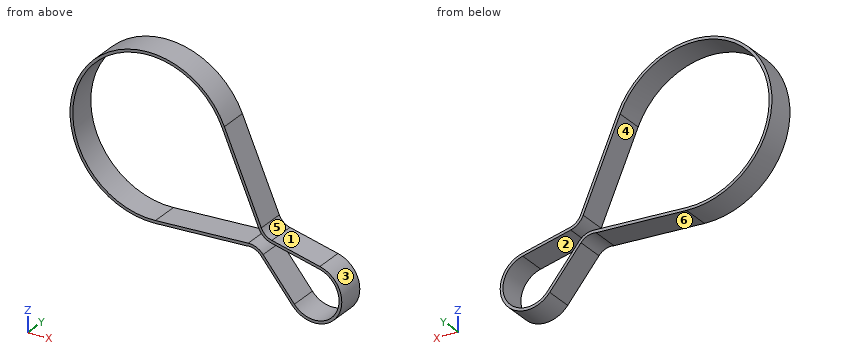
from build123d import *

# Parameters (mm, degrees)
BOSS_EXTRUDE1_DEPTH = 7
BOSS_EXTRUDE2_DEPTH = 3


with BuildPart() as part:
    # Sketch1 → Boss-Extrude1 (new body)
    with BuildSketch(Plane(origin=(0, 0, 0), x_dir=(1, 0, 0), z_dir=(0, 1, 0))):
        with BuildLine():
            Line((29.22824924, 30.681159688), (17.850659856, 16.897054356))
            ThreePointArc((17.850659856, 16.897054356), (15.379675631, 15.1910369), (12.380917697, 15.03705815))
            Line((12.380917697, 15.03705815), (-20.537634361, 17.060906053))
            ThreePointArc((-20.537634361, 17.060906053), (-47.281869491, -27.461627718), (4.525488573, -23.786335009))
            Line((4.525488573, -23.786335009), (17.958953394, 7.231589211))
            ThreePointArc((17.958953394, 7.231589211), (19.505297976, 9.287886756), (21.817685297, 10.415896524))
            Line((21.817685297, 10.415896524), (39.268754989, 14.277407445))
            ThreePointArc((39.268754989, 14.277407445), (45.745634232, 29.516516233), (29.22824924, 30.681159688))
        make_face()
        with BuildLine():
            ThreePointArc((3.607850555, -23.388917762), (-46.445589463, -26.91243355), (-20.537634361, 16.058950924))
            Line((-20.537634361, 16.058950924), (13.195989156, 13.911337267))
            ThreePointArc((13.195989156, 13.911337267), (16.191497408, 14.433261737), (18.621876492, 16.260481579))
            Line((18.621876492, 16.260481579), (29.999465876, 30.044586911))
            ThreePointArc((29.999465876, 30.044586911), (44.89272255, 28.994461003), (39.05270459, 15.253789658))
            Line((39.05270459, 15.253789658), (21.601634898, 11.392278737))
            ThreePointArc((21.601634898, 11.392278737), (18.868813518, 10.059176283), (17.041315376, 7.629006457))
            Line((17.041315376, 7.629006457), (3.607850555, -23.388917762))
        make_face(mode=Mode.SUBTRACT)
    extrude(amount=BOSS_EXTRUDE1_DEPTH)

    # Sketch2 → Boss-Extrude2 (add)
    with BuildSketch(Plane(origin=(0, 7, 0), x_dir=(1, 0, 0), z_dir=(0, 1, 0))):
        with BuildLine():
            Line((21.817685297, 10.415896524), (39.268754989, 14.277407445))
            ThreePointArc((39.268754989, 14.277407445), (45.745634232, 29.516516233), (29.22824924, 30.681159688))
            Line((29.22824924, 30.681159688), (17.850659856, 16.897054356))
            ThreePointArc((17.850659856, 16.897054356), (15.379675631, 15.1910369), (12.380917697, 15.03705815))
            Line((12.380917697, 15.03705815), (-20.537634361, 17.060906053))
            ThreePointArc((-20.537634361, 17.060906053), (-47.281869491, -27.461627718), (4.525488573, -23.786335009))
            Line((4.525488573, -23.786335009), (17.958953394, 7.231589211))
            ThreePointArc((17.958953394, 7.231589211), (19.505297976, 9.287886756), (21.817685297, 10.415896524))
        make_face()
        with BuildLine():
            Line((17.041315376, 7.629006457), (3.607850555, -23.388917762))
            ThreePointArc((3.607850555, -23.388917762), (-46.445589463, -26.91243355), (-20.537634361, 16.058950924))
            Line((-20.537634361, 16.058950924), (13.195989156, 13.911337267))
            ThreePointArc((13.195989156, 13.911337267), (16.191497408, 14.433261737), (18.621876492, 16.260481579))
            Line((18.621876492, 16.260481579), (29.999465876, 30.044586911))
            ThreePointArc((29.999465876, 30.044586911), (44.89272255, 28.994461003), (39.05270459, 15.253789658))
            Line((39.05270459, 15.253789658), (21.601634898, 11.392278737))
            ThreePointArc((21.601634898, 11.392278737), (18.868813518, 10.059176283), (17.041315376, 7.629006457))
        make_face(mode=Mode.SUBTRACT)
    extrude(amount=BOSS_EXTRUDE2_DEPTH)


solid = part.part
The listing builds one solid part. Answer for the finished solid, in the listing's coordinates (mm). Face numbers are marked on the shaded views. A direction names the side the tool comes from. Round coordinates to 2 decimals unless told otherwise and drop trailing zeros. Write each loop counter-clockwise with the first axis right and the second up, starting at its lowest first coordinate (ties: lowest second). Pieces come first, ordered by that corner, then holes. Notation, with made-up numbers: M -10,-25.5 L -2,-25.5 A19 cw -2,-13.5 Z; hole C -4,72 d6. An arc over 180 degrees is marked long. Write each question's results on one line, items separated by ' | '. Start each with the question number.
Item 1: For the marked faces 1 and 2, determine the directions among +Z, -Z, +X, -X, +Y, -Y from which every point of the face is accessible in a straight line to the end or side of a thin tool.
Item 2: A cutting plane is placed at A-A on y = 1.75. Write down the section's boundary in (x, z).
Item 3: For a pull along X with two mould halves and no side action, classify the marked faces 3, 4, 5 and 6 as pulls with the +X half, pulls with the -X half, needs draft (parallel to the pull), parting line crosses it, or undercut.
Item 4: Straight lines are drawn through the part: L1, parallel to Z at x = 29, y = 8.25; L2, parallel to X at y = 7, z = -6; L3, parallel to X at y = 5.25, z = -30.5. For each, find the intervals that lie inside material, in ascending order. Write a range as [from, to].
Item 5: A cutting plane is placed at C-C on x = 34. Write down the section's boundary in (y, z), and give its area (3 significant figures).
Item 6: A cutting plane is placed at B-B on z = 2.5. Write down the section's boundary in (x, y), and give its area (3 significant figures).
Item 7: Flat-ended cylindrical pins translate along their axes: pin 1 Ø1.5 at (y, z) = (3.5, -2.5) entering from -X; pin 2 Ø1.5 at (y, z) = (2.5, 15.5) entering from +X; pin 3 Ø1.5 at (y, z) = (8, 27.5) entering from +X. Find the tip coordinate at first contact, or state that the pin passes through.
Check sheet entries:
1) face 1: +Z, +X, +Y, -Y | face 2: +Y, -Y
2) outline: M -20.54,-17.06 L 12.38,-15.04 A5.5 cw 17.85,-16.9 L 29.23,-30.68 A10.17 ccw long 39.27,-14.28 L 21.82,-10.42 A5.5 cw 17.96,-7.23 L 4.53,23.79 A29.27 ccw long Z; hole M -20.54,-16.06 L 13.2,-13.91 A6.5 cw 18.62,-16.26 L 30,-30.04 A9.17 ccw long 39.05,-15.25 L 21.6,-11.39 A6.5 cw 17.04,-7.63 L 3.61,23.39 A28.27 ccw long Z
3) face 3: parting line crosses it | face 4: undercut | face 5: pulls with the +X half | face 6: undercut
4) L1: [-30.4, -28.83], [-13.03, -12.01] | L2: [-45.29, -44], [16.34, 17.43] | L3: [29.08, 30.4], [43.74, 45.06]
5) outline: M 0,-33.9 L 10,-33.9 L 10,-32.85 L 0,-32.85 Z; M 0,-14.14 L 10,-14.14 L 10,-13.11 L 0,-13.11 Z | area: 20.8 mm²
6) outline: M -49.97,0 L -48.9,0 L -48.9,10 L -49.97,10 Z; M 12.65,0 L 13.74,0 L 13.74,10 L 12.65,10 Z | area: 21.5 mm²
7) pin 1: x = -48.09 | pin 2: x = 8.44 | pin 3: x = 3.04
